The figure shows three views and two pictorial views of one solid part (mm, origin at its lowest corner). Answer the questions. A direction names the side the tool comes from. Coordinates: 2 decimals unless noted, no trailing zeros. Write each loop counter-clockwise with the first axis right and the second up, starting at its lowest first coordinate (ties: lowest second). Pieces come first, ordered by that corner, then holes. Notation, with made-up numbers: M -4,71.5 L 1,71.5 A24 cw 1,103.5 Z; hole C 57,-37.75 d10. An arc over 180 degrees is marked long. Use CSV: the item, a comma, the result in double quotes.
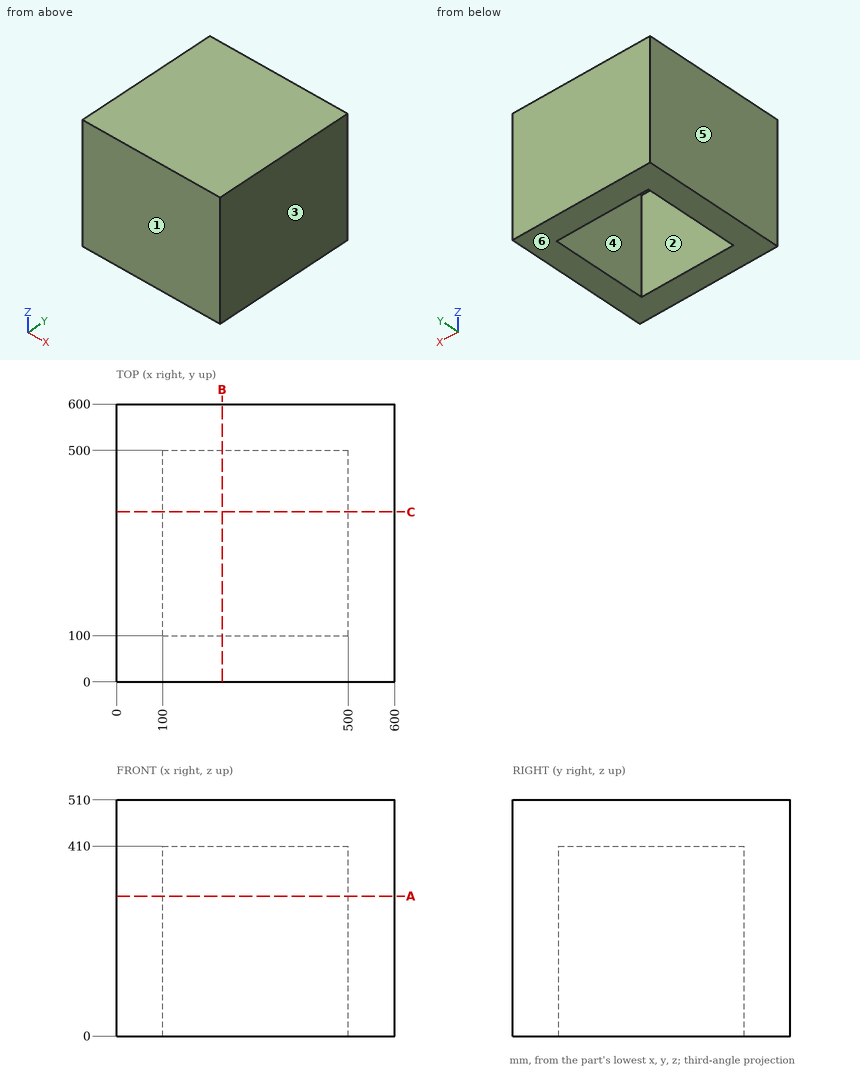
Item 1: The part is cut by section B-B (x = 227.5). Write down the section's boundary in (y, z), then the cut area to 3 significant figures.
Answer:
outline,"M 0,0 L 100,0 L 100,410 L 500,410 L 500,0 L 600,0 L 600,510 L 0,510 Z"
area,"142,000 mm2"
Item 2: The part is cut by section A-A (z = 302). Write down the section's boundary in (x, y), then the cut area to 3 significant figures.
Answer:
outline,"M 0,0 L 600,0 L 600,600 L 0,600 Z; hole M 100,100 L 500,100 L 500,500 L 100,500 Z"
area,"200,000 mm2"
Item 3: For a pull along X with two mould halves and no side action, classify the marked faces 3, 4, 5 and 6 as released by +X, released by -X, zero draft, split by the parting line, or undercut.
Answer:
face 3,"released by +X"
face 4,"undercut"
face 5,"released by -X"
face 6,"zero draft"
Item 4: A tool of negligible diameter and unlimited length cuts with its end or side. For the marked faces 1 and 2, from which of +Z, -Z, +X, -X, +Y, -Y can it reach the whole face along a straight path? Write none if from no direction.
Answer:
face 1,"+Z, -Z, +X, -X, -Y"
face 2,"-Z"
Item 5: Consider probe 1 along X at (y, z) = (362, 238.5); probe 2 along Z at (x, y) = (401, 466). Determine where each line is inside the solid, lowest interval first.
Answer:
probe 1,"x = 0 to 100, 500 to 600"
probe 2,"z = 410 to 510"
Item 6: Given pin 1 (6 mm diameter, centred on x = 327, y = 442.5, fed in from -Z), flat-ended and moving along its own axis, determine where the tip first touches the part or whether it passes through.
Answer:
pin 1,"stops at z = 410"
